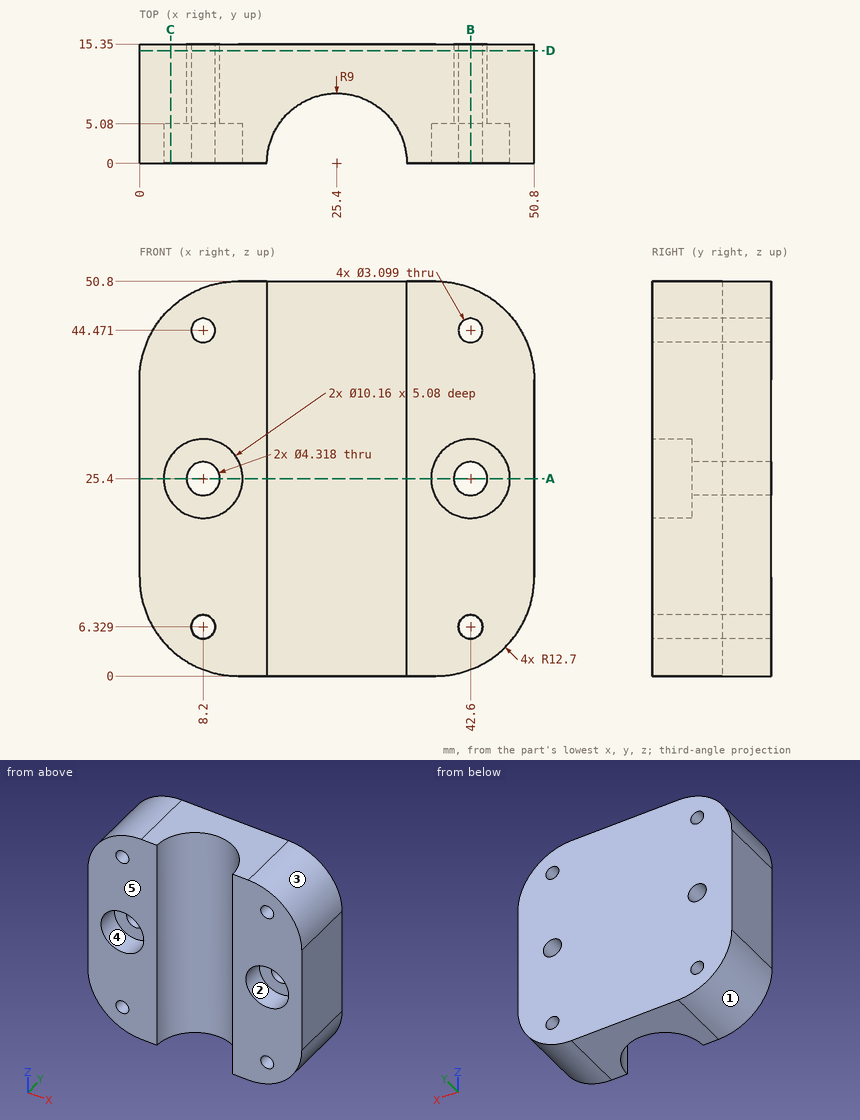
Design review of the part shown in the three views and the two pictorial views. Dimensions are in mm from the part's minimum x, y and z. A direction names the side the tool comes from. Round coordinates to 2 decimals unless told otherwise and drop trailing zeros. Loops run counter-clockwise (first coordinate to the right, second up) from the corner with the lowest first, then second, coordinate; pieces in that order, holes last. Notation, with made-up numbers: (42.5, -27) - (60.5, -27) arc R23 cw to (60.5, -3) - close; hole circle Ø2 at (24, 81.5). An arc over 180 degrees is marked (long way). Use one line per item in the form item = value.
1) We need section A-A on z = 25.4. Write out the cut boundary in (x, y).
Solutions:
outline = (0, 0) - (3.12, 0) - (3.12, 5.08) - (6.04, 5.08) - (6.04, 15.35) - (0, 15.35) - close; (10.36, 5.08) - (13.28, 5.08) - (13.28, 0) - (16.4, 0) arc R9 cw to (34.4, 0) - (37.52, 0) - (37.52, 5.08) - (40.44, 5.08) - (40.44, 15.35) - (10.36, 15.35) - close; (44.76, 5.08) - (47.68, 5.08) - (47.68, 0) - (50.8, 0) - (50.8, 15.35) - (44.76, 15.35) - close
2) Tool access review of the marked faces 1 and 2: name each direction out of +Z, -Z, +X, -X, +Y, -Y from which nothing blocks a thin tool from reaching the whole face with its end or side.
Solutions:
face_1 = -Z, -X, +Y, -Y
face_2 = -Y
3) Clearance check with flat-ended pins moving along their axes: P1, Ø1, axis at y = 3, z = 11, coming from the -X side; P2, Ø5.5, axis at x = 42.6, z = 25.4, coming from the -Y side; P3, Ø4, axis at x = 19.5, z = 10, coming from the -Y side. State where each tip first meets the part, or that it passes through.
Solutions:
P1 = 0.06
P2 = 5.08
P3 = 4.31
4) Mouldability with a two-part tool opening along X and no side actions: class the marked faces 3, 4 and 5 as pulls with the +X half, pulls with the -X half, needs draft (parallel to the pull), parting line crosses it, or undercut.
Solutions:
face_3 = pulls with the +X half
face_4 = undercut
face_5 = needs draft
5) We need section B-B on x = 42.6. Write out the cut boundary in (y, z).
Solutions:
outline = (0, 0.82) - (15.35, 0.82) - (15.35, 4.78) - (0, 4.78) - close; (0, 7.88) - (15.35, 7.88) - (15.35, 23.24) - (5.08, 23.24) - (5.08, 20.32) - (0, 20.32) - close; (0, 30.48) - (5.08, 30.48) - (5.08, 27.56) - (15.35, 27.56) - (15.35, 42.92) - (0, 42.92) - close; (0, 46.02) - (15.35, 46.02) - (15.35, 49.98) - (0, 49.98) - close
6) We need section D-D on y = 14.5. Write out the cut boundary in (x, z), then the cut area to 3 significant figures.
Solutions:
outline = (0, 12.7) arc R12.7 ccw to (12.7, 0) - (38.1, 0) arc R12.7 ccw to (50.8, 12.7) - (50.8, 38.1) arc R12.7 ccw to (38.1, 50.8) - (12.7, 50.8) arc R12.7 ccw to (0, 38.1) - close; hole circle Ø4.32 at (8.2, 25.4); hole circle Ø3.1 at (8.2, 6.33); hole circle Ø3.1 at (8.2, 44.47); hole circle Ø4.32 at (42.6, 25.4); hole circle Ø3.1 at (42.6, 6.33); hole circle Ø3.1 at (42.6, 44.47)
area = 2,380 mm2
7) We need section C-C on x = 4. Write out the cut boundary in (y, z).
Solutions:
outline = (0, 3.45) - (15.35, 3.45) - (15.35, 47.35) - (0, 47.35) - (0, 28.26) - (5.08, 28.26) - (5.08, 22.54) - (0, 22.54) - close
8) Wall thickness on probe 1 along Z at (x, y) = (8.2, 1.6) (1 decimal); probe 2 along X at (y, z) = (11, 26) (1 decimal); probe 3 along Z at (x, y) = (8.2, 8.5) (1 decimal): over which ranges is each line inside the solid? List them lowest first.
Solutions:
probe_1 = 0.8 to 4.8, 7.9 to 20.3, 30.5 to 42.9, 46 to 50
probe_2 = 0 to 6.1, 10.3 to 40.5, 44.7 to 50.8
probe_3 = 0.8 to 4.8, 7.9 to 23.2, 27.6 to 42.9, 46 to 50
